The model under review builds one solid part; all positions refer to its coordinate system, in mm. A direction names the side the tool comes from. Round coordinates to 2 decimals unless told otherwise and drop trailing zeros. Loops run counter-clockwise (first coordinate to the right, second up) from the corner with the lowest first, then second, coordinate; pieces in that order, holes last. Notation, with made-up numbers: (74.5, -15) - (82.5, -15) arc R27 ccw to (82.5, 1) - close; hole circle Ø4 at (56.5, -9). An arc over 180 degrees is marked (long way). Answer as CSV lines item,"result".
from build123d import *

# Parameters (mm, degrees)
EXTRUDE_1_DEPTH          = 20
CUT_EXTRUDE_2_DEPTH      = 40
SKETCH_4_R               = 1.5
CUT_EXTRUDE_3_DEPTH      = 40
SKETCH_5_R               = 1.5
CUT_EXTRUDE_4_DEPTH      = 40
FILLET_1_R               = 2
PATTERN_CIRCULAR_1_COUNT = 6


with BuildPart() as part:
    # 草图1 → 凸台-拉伸1 (new, symmetric)
    with BuildSketch(Plane.XY):
        with BuildLine():
            Line((0, -40), (0, -2))
            ThreePointArc((0, -2), (0.585786438, -0.585786438), (2, 0))
            Line((2, 0), (50, 0))
            Line((50, 0), (50, -1.5))
            Line((50, -1.5), (3.5, -1.5))
            ThreePointArc((3.5, -1.5), (2.085786438, -2.085786438), (1.5, -3.5))
            Line((1.5, -3.5), (1.5, -40))
            Line((1.5, -40), (0, -40))
        make_face()
    extrude(amount=EXTRUDE_1_DEPTH, both=True)

    # 草图3 → 切除-拉伸2 (cut)
    with BuildSketch(Plane.XZ.offset(1.5)):
        with BuildLine():
            Line((27, 20), (50, 20))
            Line((50, 20), (50, -20))
            Line((50, -20), (27, -20))
            ThreePointArc((27, -20), (47, 0), (27, 20))
        make_face()
        with BuildLine():
            Line((34, -6.5), (20, -6.5))
            ThreePointArc((20, -6.5), (13.5, 0), (20, 6.5))
            Line((20, 6.5), (34, 6.5))
            ThreePointArc((34, 6.5), (40.5, 0), (34, -6.5))
        make_face()
    extrude(amount=-CUT_EXTRUDE_2_DEPTH, mode=Mode.SUBTRACT)

    # 草图4 → 切除-拉伸3 (cut)
    with BuildSketch(Plane.XZ.offset(1.5)):
        with Locations(Location((27, -15.5, 0), (0, 0, 270))):
            Circle(SKETCH_4_R)
    cut_extrude_3 = extrude(amount=-CUT_EXTRUDE_3_DEPTH, mode=Mode.SUBTRACT)

    # 草图5 → 切除-拉伸4 (cut)
    with BuildSketch(Plane.ZY):
        with Locations((15, -8.5)):
            Circle(SKETCH_5_R)
        with Locations((15, -32.5)):
            Circle(SKETCH_5_R)
        with Locations((-15, -32.5)):
            Circle(SKETCH_5_R)
        with Locations((-15, -8.5)):
            Circle(SKETCH_5_R)
    extrude(amount=-CUT_EXTRUDE_4_DEPTH, mode=Mode.SUBTRACT)

    # 圆角1
    fillet_1_edges = [part.edges().sort_by_distance(p)[0] for p in [
        (0.75, -40, 20),
        (0.75, -40, -20),
    ]]
    fillet(fillet_1_edges, radius=FILLET_1_R)

    # 阵列(圆周)1: 切除-拉伸3 ×6 about axis
    pattern_circular_1_axis = Axis((27, 0, 0), (0, 1, 0))
    for i in range(1, PATTERN_CIRCULAR_1_COUNT):
        add(cut_extrude_3.rotate(pattern_circular_1_axis, i * 360 / PATTERN_CIRCULAR_1_COUNT), mode=Mode.SUBTRACT)


solid = part.part
1. Draft analysis for pull direction Y (two halves, no side actions). For faces 4 (the face through (0.7, -9.4, 13.8)), 5 (the face through (1, -10, 20)), 6 (the face through (0.74, -39.43, 19.4)), state which applies: +Y half, -Y half, draft (parallel to the pull), parting line (faces both ways), or undercut.
Numbers:
face 4,"undercut"
face 5,"draft"
face 6,"-Y half"
2. Tool access review of faces 1 (the face through (1, -40, 0)), 2 (the face through (27, -1, -6.5)), 3 (the face through (1.5, -21, 0)): name each direction out of +Z, -Z, +X, -X, +Y, -Y from which nothing blocks a thin tool from reaching the whole face with its end or side.
Numbers:
face 1,"+Z, -Z, +X, -X, -Y"
face 2,"+Y, -Y"
face 3,"+Z, -Z, +X, -Y"
3. Take a section at D-D (z = -7.75). State the section outline as (x, y) points.
Numbers:
outline,"(0, -40) - (1.5, -40) - (1.5, -3.5) arc R2 cw to (3.5, -1.5) - (12.08, -1.5) - (12.08, 0) - (2, 0) arc R2 ccw to (0, -2) - close; (15.08, -1.5) - (38.92, -1.5) - (38.92, 0) - (15.08, 0) - close; (41.92, -1.5) - (45.44, -1.5) - (45.44, 0) - (41.92, 0) - close"
4. Take a section at A-A (x = 22.5). State the section outline as (y, z) points.
Numbers:
outline,"(-1.5, -20) - (0, -20) - (0, -6.5) - (-1.5, -6.5) - close; (-1.5, 6.5) - (0, 6.5) - (0, 20) - (-1.5, 20) - close"
5. Take a section at C-C (z = 12). State the section outline as (x, y) points, plus the area to 3 significant figures.
Numbers:
outline,"(0, -40) - (1.5, -40) - (1.5, -3.5) arc R2 cw to (3.5, -1.5) - (43, -1.5) - (43, 0) - (2, 0) arc R2 ccw to (0, -2) - close"
area,"122 mm²"
6. Wall thickness on probe 1 along X at (y, z) = (-0.85, 7.75); probe 2 along Y at (x, z) = (0.85, -15); probe 3 along Y at (x, z) = (29, -17): over which ranges is each line inside the solid? List them lowest first.
Numbers:
probe 1,"x = 0.36 to 12.08, 15.08 to 38.92, 41.92 to 45.44"
probe 2,"y = -40 to -34, -31 to -10, -7 to -0.36"
probe 3,"y = -1.5 to 0"
7. Take a section at B-B (z = -15.5). State the section outline as (x, y) points.
Numbers:
outline,"(0, -40) - (1.5, -40) - (1.5, -33.91) - (0, -33.91) - close; (0, -31.09) - (1.5, -31.09) - (1.5, -9.91) - (0, -9.91) - close; (0, -7.09) - (1.5, -7.09) - (1.5, -3.5) arc R2 cw to (3.5, -1.5) - (25.5, -1.5) - (25.5, 0) - (2, 0) arc R2 ccw to (0, -2) - close; (28.5, -1.5) - (39.64, -1.5) - (39.64, 0) - (28.5, 0) - close"
8. Clearance check with flat-ended pins moving along their axes: pin 1 (2.5 mm diameter, centred on x = 27, z = 15.5, fed in from +Y); pin 2 (4 mm diameter, centred on x = 5, z = 4, fed in from -Y); pin 3 (4 mm diameter, centred on y = -32.5, z = 15, fed in from +X); pin 4 (5 mm diameter, centred on x = 13.58, z = 7.75, fed in from -Y). State where each tip first meets the part, or that it passes through.
Numbers:
pin 1,"passes through"
pin 2,"stops at y = -1.56"
pin 3,"stops at x = 1.5"
pin 4,"stops at y = -1.5"
